Answer from the drawing. Dimensions are ordinates in mm from the lowest x, y and z of the part. A direction names the side the tool comes from. Round coordinates to 2 decimals unless told otherwise and drop trailing zeros. Order: outer loops, then holes, each group sorted by start corner. A loop starts at its lowest first (then second) coordinate and runs counter-clockwise, first axis right, second up. Notation, with made-up numbers: (0, 60) -> (31, 60) arc R7 cw to (31, 66) -> close; hole circle Ø3 at (-17.5, -16.75). An arc over 180 degrees is marked (long way). Use a Markdown table: item, result. Add a question column.
Item 1: A tool of negligible diameter and unlimited length cuts with its end or side. For the marked faces 1 and 2, from which of +Z, -Z, +X, -X, +Y, -Y can it reach the whole face along a straight path? Write none if from no direction.
Item 2: Find the intervals of material crossed by L1, parallel to Y at x = 1.1, z = 1.05; L2, parallel to Z at x = 1.3, y = 12; L3, parallel to X at y = 18.75, z = 1, in increasing order. Write a range as [from, to].
Item 3: A cutting plane is placed at A-A, the plane y = 6.75. Determine the outline of the cut face in (x, z), plus the area to 3 significant figures.
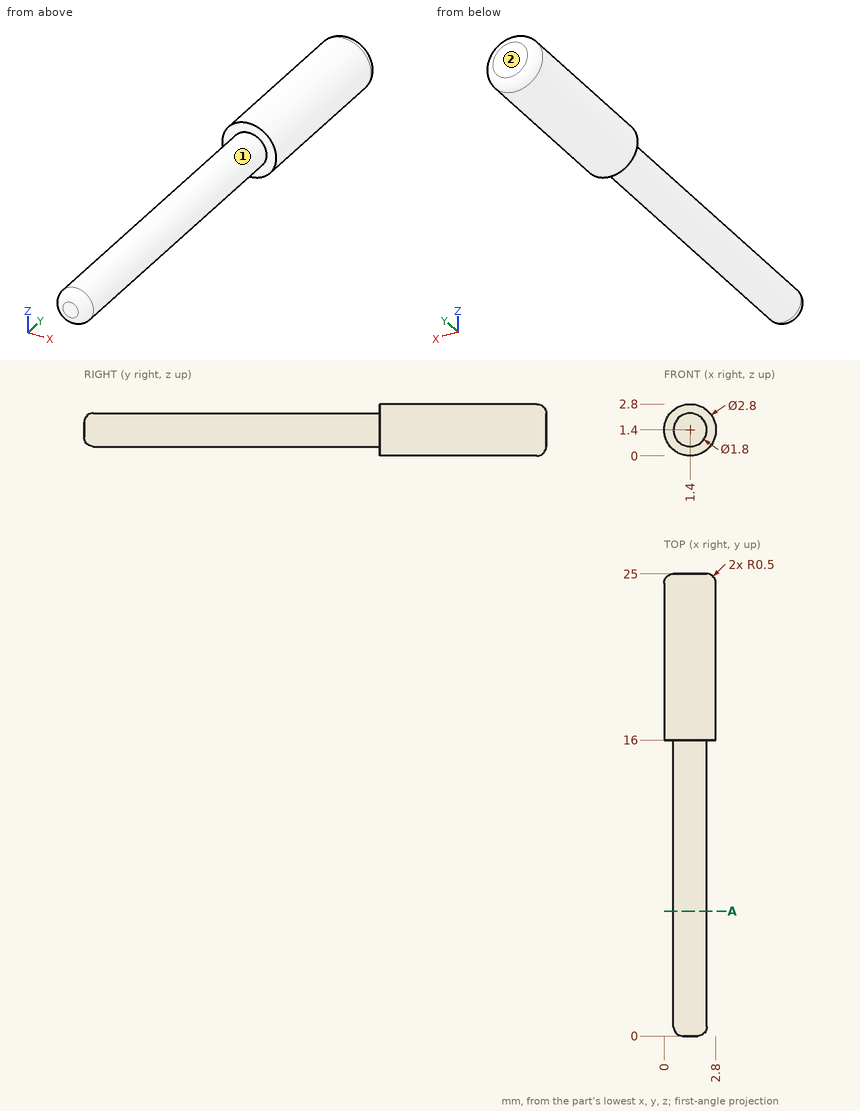
Reported:
| question | item | result |
|---|---|---|
| 1 | face 1 | -Y |
| 1 | face 2 | +Z, -Z, +X, -X, +Y |
| 2 | L1 | [0, 25] |
| 2 | L2 | [0.51, 2.29] |
| 2 | L3 | [0.06, 2.74] |
| 3 | outline | circle Ø1.8 at (1.4, 1.4) |
| 3 | area | 2.54 mm² |
